Design review of the part built by this model. Coordinates are the model's own, in mm. Round coordinates to 2 decimals unless told otherwise and drop trailing zeros. Order: outer loops, then holes, each group sorted by start corner. A loop starts at its lowest first (then second) coordinate and runs counter-clockwise, first axis right, second up. Notation, with made-up numbers: (17, -14.75) - (45, -14.75) arc R19 ccw to (45, -2.75) - close; hole circle Ø6 at (49, 61.25). An arc over 180 degrees is marked (long way). Write item = value, one per line.
from build123d import *

# Parameters (mm, degrees)
SKETCH1_W                      = 450
SKETCH1_H                      = 45
BOSS_EXTRUDE1_DEPTH            = 2
TERMINAL_12P_CUTOUT_DEPTH      = 227.131046077
TERMINAL_12P_CUTOUT_DEPTH_BACK = 227.131046077
SK_TERMINAL_12P_CUTOUT_R       = 1.625
SK_TERMINAL_12P_CUTOUT_W       = 56.92
SK_TERMINAL_12P_CUTOUT_H       = 10.9
SK_TERMINAL_12P_CUTOUT_W_2     = 34.06
SKETCH2_R                      = 2.5
CUT_EXTRUDE1_DEPTH             = 227.131046077
SKETCH3_R                      = 1.5
SKETCH3_R_2                    = 10
SKETCH3_R_3                    = 1.6
CUT_EXTRUDE2_DEPTH             = 10


with BuildPart() as part:
    # Sketch1 → Boss-Extrude1 (new body)
    with BuildSketch(Plane.XY):
        Rectangle(SKETCH1_W, SKETCH1_H)
    extrude(amount=BOSS_EXTRUDE1_DEPTH)

    # SK Terminal 12P cutout → Terminal 12P cutout (cut, two sides: drawn at the far end of the back side and taken through both)
    with BuildSketch(Plane.XY.offset(-TERMINAL_12P_CUTOUT_DEPTH_BACK)):
        with Locations((7.5, -8.35)):
            Circle(SK_TERMINAL_12P_CUTOUT_R)
        with Locations((69.67, -8.35)):
            Circle(SK_TERMINAL_12P_CUTOUT_R)
        with Locations((-46.81, -8.35)):
            Circle(SK_TERMINAL_12P_CUTOUT_R)
        with Locations((-7.5, -8.35)):
            Circle(SK_TERMINAL_12P_CUTOUT_R)
        with Locations((38.585, -8.95)):
            Rectangle(SK_TERMINAL_12P_CUTOUT_W, SK_TERMINAL_12P_CUTOUT_H)
        with Locations((-27.155, -8.95)):
            Rectangle(SK_TERMINAL_12P_CUTOUT_W_2, SK_TERMINAL_12P_CUTOUT_H)
    extrude(amount=TERMINAL_12P_CUTOUT_DEPTH + TERMINAL_12P_CUTOUT_DEPTH_BACK, mode=Mode.SUBTRACT)

    # Sketch2 → Cut-Extrude1 (cut, through all)
    with BuildSketch(Plane.XY.offset(2)):
        with Locations((-215, 0)):
            Circle(SKETCH2_R)
        with Locations((215, 0)):
            Circle(SKETCH2_R)
        with Locations((-194, 12.495407459)):
            Circle(SKETCH2_R)
        with Locations((194, 12.495407459)):
            Circle(SKETCH2_R)
        with Locations((0, 12.5)):
            Circle(SKETCH2_R)
    extrude(amount=-CUT_EXTRUDE1_DEPTH, mode=Mode.SUBTRACT)

    # Sketch3 → Cut-Extrude2 (cut)
    with BuildSketch(Plane.XY.offset(2)):
        with Locations((150, -8.55)):
            Circle(SKETCH3_R)
        with Locations((175, -8.55)):
            Circle(SKETCH3_R)
        with Locations((80, -8.55)):
            Circle(SKETCH3_R)
        with Locations((105, -8.55)):
            Circle(SKETCH3_R)
        with Locations((194, -8.55)):
            Circle(SKETCH3_R_2)
        with Locations((-194, -8.55)):
            Circle(SKETCH3_R_2)
        with Locations((-176, -8.55)):
            Circle(SKETCH3_R_3)
        with Locations((-148.5, -8.55)):
            Circle(SKETCH3_R_3)
        with BuildLine():
            Line((168.375, -14.4), (154.1, -14.4))
            ThreePointArc((154.1, -14.4), (153.392893219, -14.107106781), (153.1, -13.4))
            Line((153.1, -13.4), (153.1, -3.7))
            ThreePointArc((153.1, -3.7), (153.451471863, -2.851471863), (154.3, -2.5))
            Line((154.3, -2.5), (168.175, -2.5))
            ThreePointArc((168.175, -2.5), (170.80897276, -3.59102724), (171.9, -6.225))
            Line((171.9, -6.225), (171.9, -10.875))
            ThreePointArc((171.9, -10.875), (170.867551404, -13.367551404), (168.375, -14.4))
        make_face()
        with BuildLine():
            Line((98.375, -14.4), (84.1, -14.4))
            ThreePointArc((84.1, -14.4), (83.392893219, -14.107106781), (83.1, -13.4))
            Line((83.1, -13.4), (83.1, -3.7))
            ThreePointArc((83.1, -3.7), (83.451471863, -2.851471863), (84.3, -2.5))
            Line((84.3, -2.5), (98.175, -2.5))
            ThreePointArc((98.175, -2.5), (100.80897276, -3.59102724), (101.9, -6.225))
            Line((101.9, -6.225), (101.9, -10.875))
            ThreePointArc((101.9, -10.875), (100.867551404, -13.367551404), (98.375, -14.4))
        make_face()
        with BuildLine():
            Line((-171, -19.05), (-153.5, -19.05))
            ThreePointArc((-153.5, -19.05), (-152.085786438, -18.464213562), (-151.5, -17.05))
            Line((-151.5, -17.05), (-151.5, -0.05))
            ThreePointArc((-151.5, -0.05), (-152.085786438, 1.364213562), (-153.5, 1.95))
            Line((-153.5, 1.95), (-171, 1.95))
            ThreePointArc((-171, 1.95), (-172.414213562, 1.364213562), (-173, -0.05))
            Line((-173, -0.05), (-173, -17.05))
            ThreePointArc((-173, -17.05), (-172.414213562, -18.464213562), (-171, -19.05))
        make_face()
    extrude(amount=-CUT_EXTRUDE2_DEPTH, mode=Mode.SUBTRACT)


solid = part.part
Item 1: Take a section at B-B, the plane z = 0.5. Count the separate pieces of the cut face and the enclosed holes in it, and give its area (3 significant figures).
Data:
separate_pieces = 1
enclosed_holes = 22
area = 17,600 mm2
Item 2: For line 1 along Y through (x, z) = (-194, 0.8); line 2 along X through (y, z) = (2, 1.25); line 3 along Y through (x, z) = (80, 1.1), list the stretches that pass through material, from the lowest coordinate up. Write a range as [from, to].
Data:
line_1 = [-22.5, -18.55], [1.45, 10], [15, 22.5]
line_2 = [-225, -216.5], [-213.5, 213.5], [216.5, 225]
line_3 = [-22.5, -10.05], [-7.05, 22.5]
Item 3: Insertion check: P1, Ø3.5, axis at x = -176, y = -8.55, coming from the +Z side. The pin has a flat end and moves straight along its axis. Give the tip position at first contact, or say it passes through.
Data:
P1 = 2
Item 4: Take a section at A-A, the plane x = 47.5. State the section outline as (y, z) points.
Data:
outline = (-22.5, 0) - (-14.4, 0) - (-14.4, 2) - (-22.5, 2) - close; (-3.5, 0) - (22.5, 0) - (22.5, 2) - (-3.5, 2) - close
Item 5: The part is to be moulded in two halves that separate along X. For faces 1 (the face through (203.237, -12.38, 1.014)), 2 (the face through (-184.763, -12.38, 1.014)), 3 (the face through (-3, 0, 0)), say which applies: +X half, -X half, draft (parallel to the pull), parting line (faces both ways), or undercut.
Data:
face_1 = undercut
face_2 = undercut
face_3 = draft
